Part model, mm, in its own coordinate system. Face numbers are marked on the shaded views. A direction names the side the tool comes from. Give positions to 0.01 mm unless a question says otherwise; leave off trailing zeros. Order: outer loops, then holes, each group sorted by start corner. A loop starts at its lowest first (then second) coordinate and runs counter-clockwise, first axis right, second up. Notation, with made-up numbers: (-39, 34.5) - (13, 34.5) arc R32 cw to (13, 73.5) - close; hole circle Ø4 at (1, -1.75). An arc over 180 degrees is marked (long way). Use one line per item in the form item = value. Start each with the question number.
1. Band-saw the part on D-D, the plane x = 37.5. List the corners of the cut face in (y, z), plus the area to 3 significant figures.
2. Drill centre lines: line 1 (X direction, y = 16.75, z = 1.5); line 2 (Z direction, x = 20, y = 13); line 3 (Z direction, x = 36.5, y = 2.25). Where is each one in solid material? Low to high.
3. Tool access for the marked faces 4, 5, 6, 7 and 8: list every direction of +Z, -Z, +X, -X, +Y, -Y with a clear straight run to the whole face (end or side of a thin tool).
4. Band-saw the part on B-B, the plane x = 26.5. List the corners of the cut face in (y, z) (3 decimals).
5. Pin check, flat tips, straight feed: P1, Ø6, axis at y = 15.5, z = 14, coming from the +X side; P2, Ø8, axis at x = 32.5, z = 16.5, coming from the -Y side; P3, Ø0.9, axis at y = 8, z = 4, coming from the -X side. Stop position of each tip, or through.
6. Pull direction Z, two halves, no side cores. Call the marked faces 1, 2 and 3: +Z half, -Z half, draft (parallel to the pull), parting line (faces both ways), or undercut.
7. Band-saw the part on A-A, the plane z = 3.5. List the corners of the cut face in (x, y).
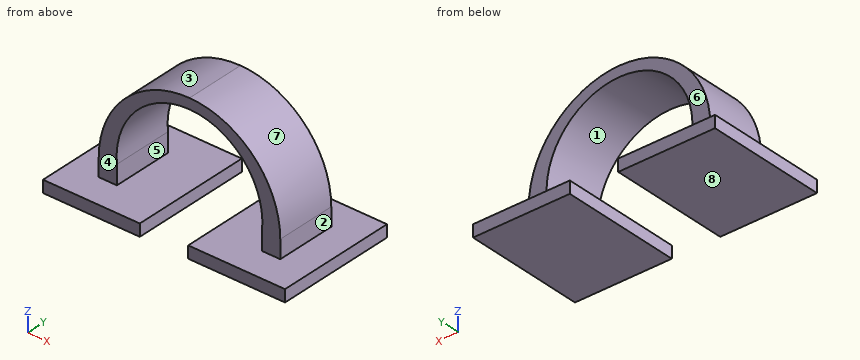
Autodesk Fusion 360 part; units mm, degrees
sketch "Sketch1" plane through (0, 0, 0) normal (0, 0, 1) x (1, 0, 0)
  line L0 (0, 0) -> (40, 0)
  line L1 (40, 0) -> (40, 20)
  line L2 (40, 20) -> (0, 20)
  line L3 (0, 20) -> (0, 0)
  line L4 (5, 15) -> (35, 15)
  line L5 (35, 15) -> (35, 5)
  line L6 (35, 5) -> (5, 5)
  line L7 (5, 5) -> (5, 15)
  line L8 (16, 0) -> (16, 20)
  line L9 (24, 0) -> (24, 20)
  dimension "d1" = 40
  dimension "d2" = 20
  dimension "d3" = 5
  dimension "d4" = 5
  dimension "d5" = 10
  dimension "d6" = 5
  dimension "d16" = 16
  dimension "d17" = 8
extrude "Extrude1" add sketch "Sketch1" along normal blind 2
extrude "Extrude2" add sketch "Sketch1" along normal blind 20 contours L4 L6 L8 L9 | L4 L6 L7 L8 | L4 L5 L6 L9
fillet "Fillet1" radius 15 2 edges at (5, 10, 20) (35, 10, 20)
sketch "Sketch2" plane through (0, 5, 0) normal (0, -1, 0) x (1, 0, 0)
  arc A0 (35, 5) -> (5, 5) centre (20, 5) ccw
  line L0 (5, 5) -> (5, 2)
  line L1 (5, 2) -> (35, 2)
  line L2 (35, 2) -> (35, 5)
  line L3 (8, 5.1637) -> (32, 5.1637)
  arc A1 (32, 5.1637) -> (8, 5.1637) centre (20, 6.2496) ccw
  line L4 (8, 5.1637) -> (8, 2)
  line L5 (32, 5.1637) -> (32, 2)
  line L6 (8, 2) -> (32, 2)
  dimension "d13" = 3
  dimension "d14" = 3
extrude "Extrude3" cut sketch "Sketch2" against normal through all contours L1 L3 L4 L5 L6 | L3 A1
extrude "Extrude4" cut sketch "Sketch1" along normal blind 2 contours L0 L6 L8 L9 | L4 L6 L8 L9 | L2 L4 L8 L9
From the geometry:
q1.outline = (0, 0) - (20, 0) - (20, 2) - (0, 2) - close
q1.area = 40.0 mm²
q2.line_1 = 0 to 16, 24 to 40
q2.line_2 = 18.3 to 20
q2.line_3 = 0 to 2
q3.face_4 = +Z, +X, -X, -Y
q3.face_5 = +Y, -Y
q3.face_6 = +Z, +X, -X, +Y
q3.face_7 = +Z, +X, +Y, -Y
q3.face_8 = -Z, +X, -X, +Y, -Y
q4.outline = (0, 0) - (20, 0) - (20, 2) - (0, 2) - close; (5, 16.395) - (15, 16.395) - (15, 18.52) - (5, 18.52) - close
q5.P1 = 33.73
q5.P2 = 5
q5.P3 = 5
q6.face_1 = undercut
q6.face_2 = draft
q6.face_3 = +Z half
q7.outline = (5, 5) - (8, 5) - (8, 15) - (5, 15) - close; (32, 5) - (35, 5) - (35, 15) - (32, 15) - close
